```python
from build123d import *

# Parameters (mm, degrees)
F0_R      = 5
F0_W      = 15
F0_H      = 14
F1_DEPTH  = 3
F0_W_2    = 5
F0_H_2    = 23
F2_DEPTH  = 1
F0_R_2    = 1.4
F3_DEPTH  = 15.5
F4_DEPTH  = 3
F5_R      = 2
F6_W      = 7.25
F6_H      = 4
F7_DEPTH  = 25
F8_W      = 8.5
F8_H      = 3.25
F9_DEPTH  = 25
F8_W_2    = 11.5
F8_H_2    = 6.25
F10_DEPTH = 1
F11_R     = 2
F12_DEPTH = 2
F13_SIZE  = 2.99999


# Not quite as in the source:
# - a fillet or chamfer is up to 0.001 mm smaller than in the source, because OpenCascade refuses the exact size
# - a feature names something its author has since deleted; it is built from what else it names


with BuildPart() as f1:
    # F0 (on Top) → F1 (new body)
    with BuildSketch(Plane.XY):
        with BuildLine():
            ThreePointArc((35.5, 21.1314561435), (31.3079689783, 21.3079689783), (31.1314561435, 25.5))
            Line((31.1314561435, 25.5), (-31.1314561435, 25.5))
            ThreePointArc((-31.1314561435, 25.5), (-31.3079689783, 21.3079689783), (-35.5, 21.1314561435))
            Line((-35.5, 21.1314561435), (-35.5, -21.1314561435))
            ThreePointArc((-35.5, -21.1314561435), (-31.3079689783, -21.3079689783), (-31.1314561435, -25.5))
            Line((-31.1314561435, -25.5), (31.1314561435, -25.5))
            ThreePointArc((31.1314561435, -25.5), (31.3079689783, -21.3079689783), (35.5, -21.1314561435))
            Line((35.5, -21.1314561435), (35.5, 21.1314561435))
        make_face()
        with Locations((-21.7, 0)):
            Circle(F0_R, mode=Mode.SUBTRACT)
        with Locations((-21.8, 13.25)):
            Rectangle(F0_W, F0_H, mode=Mode.SUBTRACT)
        Polygon((-7.6, -20.25), (-7.6, 20.25), (27, 20.25), (27, 11.5), (32, 11.5), (32, -11.5), (27, -11.5), (27, -20.25), align=None, mode=Mode.SUBTRACT)
    extrude(amount=F1_DEPTH)

    # F0 (on Top) → F2 (join)
    with BuildSketch(Plane.XY):
        with Locations((29.5, 0)):
            Rectangle(F0_W_2, F0_H_2)
    extrude(amount=F2_DEPTH)

    # F0 (on Top) → F3 (join)
    with BuildSketch(Plane.XY):
        with BuildLine():
            ThreePointArc((37.5, 25.5), (36.9142135624, 26.9142135624), (35.5, 27.5))
            Line((35.5, 27.5), (-35.5, 27.5))
            ThreePointArc((-35.5, 27.5), (-36.9142135624, 26.9142135624), (-37.5, 25.5))
            Line((-37.5, 25.5), (-37.5, -25.5))
            ThreePointArc((-37.5, -25.5), (-36.9142135624, -26.9142135624), (-35.5, -27.5))
            Line((-35.5, -27.5), (35.5, -27.5))
            ThreePointArc((35.5, -27.5), (36.9142135624, -26.9142135624), (37.5, -25.5))
            Line((37.5, -25.5), (37.5, 25.5))
        make_face()
        Polygon((31.1314561435, 25.5), (35.5, 25.5), (35.5, 21.1314561435), (35.5, -21.1314561435), (35.5, -25.5), (31.1314561435, -25.5), (-31.1314561435, -25.5), (-35.5, -25.5), (-35.5, -21.1314561435), (-35.5, 21.1314561435), (-35.5, 25.5), (-31.1314561435, 25.5), align=None, mode=Mode.SUBTRACT)
        with BuildLine():
            ThreePointArc((-35.5, 21.1314561435), (-31.3079689783, 21.3079689783), (-31.1314561435, 25.5))
            Line((-31.1314561435, 25.5), (-35.5, 25.5))
            Line((-35.5, 25.5), (-35.5, 21.1314561435))
        make_face()
        with Locations((-33.5, 23.5)):
            Circle(F0_R_2, mode=Mode.SUBTRACT)
        with BuildLine():
            ThreePointArc((-31.1314561435, -25.5), (-31.3079689783, -21.3079689783), (-35.5, -21.1314561435))
            Line((-35.5, -21.1314561435), (-35.5, -25.5))
            Line((-35.5, -25.5), (-31.1314561435, -25.5))
        make_face()
        with Locations((-33.5, -23.5)):
            Circle(F0_R_2, mode=Mode.SUBTRACT)
        with BuildLine():
            Line((35.5, -25.5), (35.5, -21.1314561435))
            ThreePointArc((35.5, -21.1314561435), (31.3079689783, -21.3079689783), (31.1314561435, -25.5))
            Line((31.1314561435, -25.5), (35.5, -25.5))
        make_face()
        with Locations((33.5, -23.5)):
            Circle(F0_R_2, mode=Mode.SUBTRACT)
        with BuildLine():
            Line((35.5, 21.1314561435), (35.5, 25.5))
            Line((35.5, 25.5), (31.1314561435, 25.5))
            ThreePointArc((31.1314561435, 25.5), (31.3079689783, 21.3079689783), (35.5, 21.1314561435))
        make_face()
        with Locations((33.5, 23.5)):
            Circle(F0_R_2, mode=Mode.SUBTRACT)
    extrude(amount=F3_DEPTH)

    # F0 (on Top) → F4 (join)
    with BuildSketch(Plane.XY):
        with Locations((33.5, -23.5)):
            Circle(F0_R_2)
        with Locations((33.5, 23.5)):
            Circle(F0_R_2)
        with Locations((-33.5, 23.5)):
            Circle(F0_R_2)
        with Locations((-33.5, -23.5)):
            Circle(F0_R_2)
    extrude(amount=F4_DEPTH)

    # F5
    f5_edges = [f1.edges().sort_by_distance(p)[0] for p in [
        (-37.5, 0, 0),
    ]]
    fillet(f5_edges, radius=F5_R)

    # F6 (on face) → F7 (cut)
    with BuildSketch(Plane(origin=(0, 27.5, 0), x_dir=(-1, 0, 0), z_dir=(0, 1, 0))):
        with Locations((5.3, 9.6)):
            Rectangle(F6_W, F6_H)
    extrude(amount=-F7_DEPTH, mode=Mode.SUBTRACT)

    # F8 (on face) → F9 (cut)
    with BuildSketch(Plane.XZ.offset(27.5)):
        with Locations((-6.25, 10.075)):
            Rectangle(F8_W, F8_H)
    extrude(amount=-F9_DEPTH, mode=Mode.SUBTRACT)

    # F8 (on face) → F10 (cut)
    with BuildSketch(Plane.XZ.offset(27.5)):
        with Locations((-6.25, 10.075)):
            Rectangle(F8_W_2, F8_H_2)
        with Locations((-6.25, 10.075)):
            Rectangle(F8_W, F8_H, mode=Mode.SUBTRACT)
    extrude(amount=-F10_DEPTH, mode=Mode.SUBTRACT)

    # F11
    f11_edges = [f1.edges().sort_by_distance(p)[0] for p in [
        (-0.5, -27, 13.2),
        (-0.5, -27, 6.95),
        (-12, -27, 6.95),
        (-12, -27, 13.2),
    ]]
    fillet(f11_edges, radius=F11_R)

    # F0 (on Top) → F12 (join)
    with BuildSketch(Plane.XY):
        with Locations((-21.8, 13.25)):
            Rectangle(F0_W, F0_H)
    extrude(amount=F12_DEPTH)

    # F13 (size 3 in the source; OpenCascade refuses exactly that, so slightly less here)
    f13_edges = [f1.edges().sort_by_distance(p)[0] for p in [
        (-26.7, 0, 0),
    ]]
    chamfer(f13_edges, length=F13_SIZE)


solid = f1.part
```
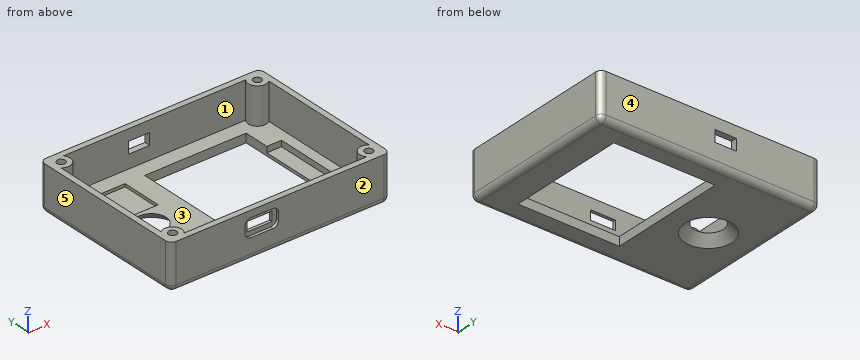
Read the model definition and answer for the solid it produces. Units are mm, in the model's axes. Face numbers are marked on the shaded views. A direction names the side the tool comes from. Coordinates: 2 decimals unless noted, no trailing zeros. Loops run counter-clockwise (first coordinate to the right, second up) from the corner with the lowest first, then second, coordinate; pieces in that order, holes last. Notation, with made-up numbers: (-20.5, 35.5) - (8.5, 35.5) arc R22 cw to (8.5, 65.5) - close; hole circle Ø4 at (54, -30). An arc over 180 degrees is marked (long way). Answer in a Markdown table with one row per item.
1. Which of the six approach directions +Z, -Z, +X, -X, +Y, -Y give full straight-line access (tool end or side, diameter ignored) to the marked faces 1 and 2?
Conclusion:
| item | result |
|---|---|
| face 1 | +Z |
| face 2 | +Z, -Z, +X, -X, -Y |
2. Given pin 1 (1.5 mm diameter, centred on y = -8.5, z = 1, fed in from +X); pin 2 (1.5 mm diameter, centred on x = 18, z = 1, fed in from -Y); pin 3 (2 mm diameter, centred on x = -15, y = 17.5, fed in from +Z), each flat-ended and moving along its own axis, determine where each tip first touches the part or whether it passes through.
Conclusion:
| item | result |
|---|---|
| pin 1 | stops at x = 37.48 |
| pin 2 | stops at y = -27.48 |
| pin 3 | stops at z = 3 |
3. Find section C-C, the plane y = 0. Count the separate pieces of the cut face and the enclosed holes in it, then the cut area to 3 significant figures.
Conclusion:
| item | result |
|---|---|
| separate pieces | 3 |
| enclosed holes | 0 |
| area | 120 mm² |
4. Straight lines are drawn through the part: line 1 (Y direction, x = -33.5, z = 9); line 2 (Y direction, x = -21.7, z = 3.05); line 3 (X direction, y = -2.5, z = 3.75). For each, find the intervals that lie inside material, in ascending order.
Conclusion:
| item | result |
|---|---|
| line 1 | y = -27.5 to -24.9, -22.1 to -20.4, 20.4 to 22.1, 24.9 to 27.5 |
| line 2 | y = -27.5 to -25.5, 25.5 to 27.5 |
| line 3 | x = -37.5 to -35.5, 35.5 to 37.5 |
5. Find section D-D, the plane y = -23.5. Write down the section's boundary in (x, z), then the cut area to 3 significant figures.
Conclusion:
| item | result |
|---|---|
| outline | (-37.5, 2) arc R2 ccw to (-35.5, 0) - (35.5, 0) arc R2 ccw to (37.5, 2) - (37.5, 15.5) - (34.9, 15.5) - (34.9, 3) - (32.1, 3) - (32.1, 15.5) - (30.4, 15.5) - (30.4, 3) - (-30.4, 3) - (-30.4, 15.5) - (-32.1, 15.5) - (-32.1, 3) - (-34.9, 3) - (-34.9, 15.5) - (-37.5, 15.5) - close |
| area | 331 mm² |
6. Determine the mould class of the marked faces 3, 4 and 5 for opening direction X: +X half, -X half, draft (parallel to the pull), parting line (faces both ways), or undercut.
Conclusion:
| item | result |
|---|---|
| face 3 | undercut |
| face 4 | draft |
| face 5 | -X half |
7. Find section A-A, the plane y = 14. Write down the section's boundary in (x, z), then the cut area to 3 significant figures.
Conclusion:
| item | result |
|---|---|
| outline | (-37.5, 2) arc R2 ccw to (-35.5, 0) - (-7.6, 0) - (-7.6, 3) - (-14.3, 3) - (-14.3, 2) - (-29.3, 2) - (-29.3, 3) - (-35.5, 3) - (-35.5, 15.5) - (-37.5, 15.5) - close; (27, 0) - (35.5, 0) arc R2 ccw to (37.5, 2) - (37.5, 15.5) - (35.5, 15.5) - (35.5, 3) - (27, 3) - close |
| area | 154 mm² |
